```python
from build123d import *

# Parameters (mm, degrees)
F4_R     = 15.875
F5_DEPTH = 76.2


# Not quite as in the source:
# - a feature of the source that left no trace in its solid (it failed there, or was rolled back) is left out


with BuildPart() as f1:
    # F0 (on Front) → F1 (revolve)
    with BuildSketch(Plane.XZ):
        Polygon((0, -22.6070340723), (0, 0), (47.3772140821, 59.6811493339), (40.7688170671, 59.6811493339), (-6.0150707141, 0), (-25.4921261221, 0), (-25.4921261221, -22.6070340723), align=None)
    revolve(axis=Axis((-25.4921261221, 0, -11.3035170361), (0, 0, -1)))

    # F4 (on face) → F5 (cut)
    with BuildSketch(Plane.XY):
        with Locations((-25.4921261221, 0)):
            Circle(F4_R)
    extrude(amount=-F5_DEPTH, mode=Mode.SUBTRACT)


solid = f1.part
```
The listing builds one solid part. Answer for the finished solid, in the listing's coordinates (mm). A direction names the side the tool comes from. Give positions to 0.01 mm unless a question says otherwise; leave off trailing zeros. Order: outer loops, then holes, each group sorted by start corner. A loop starts at its lowest first (then second) coordinate and runs counter-clockwise, first axis right, second up.
1) For faces 1 (the face through (-32.8, 14.3, 0)), 2 (the face through (-50.96, -1.12, -11.15)), 3 (the face through (-10.828, -6.08, -11.145)), determine the directions among +Z, -Z, +X, -X, +Y, -Y from which every point of the face is accessible in a straight line to the end or side of a thin tool.
Reported:
face 1: +Z
face 2: -Z
face 3: +Z, -Z
2) Given P1, Ø1, axis at x = -62.5, y = 27.5, coming from the +Z side; P2, Ø1, axis at x = -49.5, y = 42, coming from the -Z side; P3, Ø4, axis at x = -78, y = 7.5, coming from the +Z side, each flat-ended and moving along its own axis, determine where each tip first touches the part or whether it passes through.
Reported:
P1: stops at z = 34.61
P2: stops at z = 28.2
P3: stops at z = 45.37
3) Find section A-A on y = 0. Write down the section's boundary in (x, z).
Reported:
outline: (-98.36, 59.68) - (-50.98, 0) - (-50.98, -22.61) - (-41.37, -22.61) - (-41.37, 0) - (-44.97, 0) - (-91.75, 59.68) - close; (-9.62, -22.61) - (0, -22.61) - (0, 0) - (47.38, 59.68) - (40.77, 59.68) - (-6.02, 0) - (-9.62, 0) - close
4) Consider line 1 along Y through (x, z) = (-26, -2); line 2 along X through (y, z) = (9, 17); line 3 along Y through (x, z) = (-27, 13). Determine where each line is inside the solid, lowest interval first.
Reported:
line 1: y = -25.49 to -15.87, 15.87 to 25.49
line 2: x = -63.43 to -57.04, 6.05 to 12.44
line 3: y = -35.78 to -29.63, 29.63 to 35.78
5) Determine the mould class of faces 4 (the face through (1.65, -8.547, 3.733)), 5 (the face through (-42, 64.4, 59.681)), 6 (the face through (-46.876, 16.397, 9.529)) for opening direction X: pulls with the +X half, pulls with the -X half, needs draft (parallel to the pull), parting line crosses it, or undercut.
Reported:
face 4: parting line crosses it
face 5: needs draft
face 6: undercut
6) Find section C-C on z = 12.5. Write down the section's boundary in (x, y), then the cut area to 3 significant figures.
Reported:
outline: circle Ø70.83 at (-25.49, 0); hole circle Ø58.55 at (-25.49, 0)
area: 1,250 mm2
7) Find section B-B on z = -16. Write down the section's boundary in (x, y) (3 decimals).
Reported:
outline: circle Ø50.984 at (-25.492, 0); hole circle Ø31.75 at (-25.492, 0)
